The model under review builds one solid part; all positions refer to its coordinate system, in mm. Give positions to 0.01 mm unless a question says otherwise; leave off trailing zeros. Order: outer loops, then holes, each group sorted by start corner. A loop starts at its lowest first (then second) coordinate and runs counter-clockwise, first axis right, second up. Notation, with made-up numbers: (42, 31.25) - (48, 31.25) arc R25 ccw to (48, 44.25) - close; hole circle Ø1 at (33.25, 69.5). An arc over 180 degrees is marked (long way). Use CSV: the item, a comma, the result in double quotes.
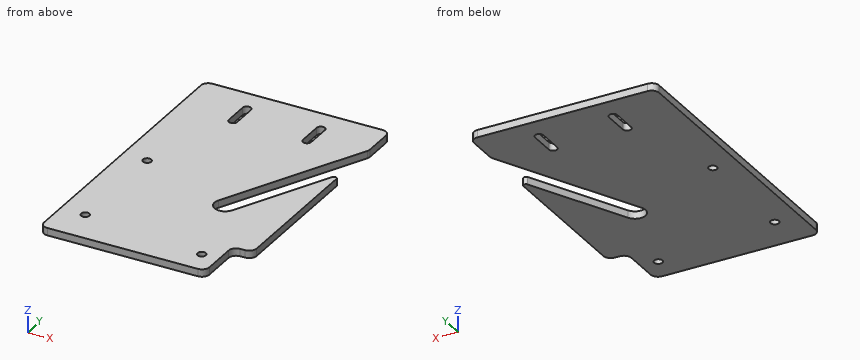
```python
from build123d import *

# Parameters (mm, degrees)
SKETCH1_R           = 1.7
BOSS_EXTRUDE1_DEPTH = 3
FILLET1_R           = 3
CUT_EXTRUDE1_DEPTH  = 4
SKETCH3_W           = 8
SKETCH3_H           = 20
CUT_EXTRUDE2_DEPTH  = 4
FILLET2_R           = 3
FILLET3_R           = 1


with BuildPart() as part:
    # Sketch1 → Boss-Extrude1 (new body)
    with BuildSketch(Plane.XY):
        with BuildLine():
            Line((75, 0), (0, 0))
            Line((0, 0), (0, -120))
            Line((0, -120), (75, -120))
            Line((75, -120), (75, -34.726895702))
            Line((75, -34.726895702), (63.890758281, -56.94537914))
            Line((63.890758281, -56.94537914), (53.890758281, -76.94537914))
            ThreePointArc((53.890758281, -76.94537914), (48.05462086, -78.890758281), (46.109241719, -73.05462086))
            Line((46.109241719, -73.05462086), (56.109241719, -53.05462086))
            Line((56.109241719, -53.05462086), (75, -15.273104298))
            Line((75, -15.273104298), (75, 0))
        make_face()
        with Locations((10, -105)):
            Circle(SKETCH1_R, mode=Mode.SUBTRACT)
        with Locations((60, -110)):
            Circle(SKETCH1_R, mode=Mode.SUBTRACT)
        with Locations((10, -60)):
            Circle(SKETCH1_R, mode=Mode.SUBTRACT)
    extrude(amount=BOSS_EXTRUDE1_DEPTH)

    # Fillet1
    fillet1_edges = [part.edges().sort_by_distance(p)[0] for p in [
        (75, -120, 1.5),
        (0, -120, 1.5),
        (0, 0, 1.5),
        (75, 0, 1.5),
        (75, -15.273104298, 1.5),
    ]]
    fillet(fillet1_edges, radius=FILLET1_R)

    # Sketch2 → Cut-Extrude1 (cut, through all)
    with BuildSketch(Plane.XY.offset(3)):
        with BuildLine():
            Line((20.8, -10), (20.8, -20))
            ThreePointArc((20.8, -20), (22.5, -21.7), (24.2, -20))
            Line((24.2, -20), (24.2, -10))
            ThreePointArc((24.2, -10), (22.5, -8.3), (20.8, -10))
        make_face()
        with BuildLine():
            Line((50.8, -10), (50.8, -20))
            ThreePointArc((50.8, -20), (52.5, -21.7), (54.2, -20))
            Line((54.2, -20), (54.2, -10))
            ThreePointArc((54.2, -10), (52.5, -8.3), (50.8, -10))
        make_face()
    extrude(amount=-CUT_EXTRUDE1_DEPTH, mode=Mode.SUBTRACT)

    # Sketch3 → Cut-Extrude2 (cut, through all)
    with BuildSketch(Plane.XY.offset(3)):
        with Locations((71, -110)):
            Rectangle(SKETCH3_W, SKETCH3_H)
    extrude(amount=-CUT_EXTRUDE2_DEPTH, mode=Mode.SUBTRACT)

    # Fillet2
    fillet2_edges = [part.edges().sort_by_distance(p)[0] for p in [
        (75, -100, 1.5),
        (67, -120, 1.5),
        (67, -100, 1.5),
    ]]
    fillet(fillet2_edges, radius=FILLET2_R)

    # Fillet3
    fillet3_edges = [part.edges().sort_by_distance(p)[0] for p in [
        (75, -34.726895702, 1.5),
    ]]
    fillet(fillet3_edges, radius=FILLET3_R)


solid = part.part
```
Item 1: Take a section at D-D, the plane z = 2. State how many separate pieces and enclosed holes the cut face has, and give its area (3 significant figures).
Results list:
separate pieces,"1"
enclosed holes,"5"
area,"8,200 mm2"
Item 2: Wall thickness on L1, parallel to Y at x = 10, z = 1.15; L2, parallel to Y at x = 60, z = 1.75; L3, parallel to X at y = -105, z = 1.45: over which ranges is each line inside the solid? List them lowest first.
Results list:
L1,"y = -120 to -106.7, -103.3 to -61.7, -58.3 to 0"
L2,"y = -120 to -111.7, -108.3 to -64.73, -45.27 to 0"
L3,"x = 0 to 8.3, 11.7 to 67"
Item 3: Take a section at C-C, the plane y = -105. Give the boundary of the cut face in (x, z), and give its area (3 significant figures).
Results list:
outline,"(0, 0) - (8.3, 0) - (8.3, 3) - (0, 3) - close; (11.7, 0) - (67, 0) - (67, 3) - (11.7, 3) - close"
area,"191 mm2"
Item 4: Clearance check with flat-ended pins moving along their axes: pin 1 (2.5 mm diameter, centred on x = 60, y = -110, fed in from -Z); pin 2 (0.9 mm diameter, centred on y = -109, z = 2, fed in from +X); pin 3 (0.6 mm diameter, centred on x = 71.5, z = 1.5, fed in from -Y). State where each tip first meets the part, or that it passes through.
Results list:
pin 1,"passes through"
pin 2,"stops at x = 67"
pin 3,"stops at y = -100"
Item 5: Take a section at B-B, the plane y = -11.5. Give the boundary of the cut face in (x, z), and give its area (3 significant figures).
Results list:
outline,"(0, 0) - (20.8, 0) - (20.8, 3) - (0, 3) - close; (24.2, 0) - (50.8, 0) - (50.8, 3) - (24.2, 3) - close; (54.2, 0) - (75, 0) - (75, 3) - (54.2, 3) - close"
area,"205 mm2"
Item 6: Take a section at A-A, the plane x = 22.5. Give the boundary of the cut face in (y, z).
Results list:
outline,"(-120, 0) - (-21.7, 0) - (-21.7, 3) - (-120, 3) - close; (-8.3, 0) - (0, 0) - (0, 3) - (-8.3, 3) - close"
